```python
from build123d import *

# Parameters (mm, degrees)
F0_W     = 41
F0_H     = 106
F0_R     = 1.5
F0_R_2   = 5.05
F0_R_3   = 2
F0_R_4   = 3
F0_R_5   = 9.5
F1_DEPTH = 3
F2_R     = 3


# Not quite as in the source:
# - a feature names something its author has since deleted; it is built from what else it names


with BuildPart() as f1:
    # F0 (on Top) → F1 (new body)
    with BuildSketch(Plane.XY):
        with Locations((-1.1801278293, -1.1353523731)):
            Rectangle(F0_W, F0_H)
        with Locations((-18.2301278293, -51.4703523731)):
            Circle(F0_R, mode=Mode.SUBTRACT)
        with Locations((-6.776117335, -33.481924504)):
            Circle(F0_R_2, mode=Mode.SUBTRACT)
        with Locations((-18.2301278293, -21.2703523731)):
            Circle(F0_R, mode=Mode.SUBTRACT)
        with Locations((-11.8353097141, -18.4490393624)):
            Circle(F0_R_3, mode=Mode.SUBTRACT)
        with BuildLine():
            ThreePointArc((0.9913514778, -28.481924504), (-4.9415118708, -25.855220261), (-8.0481067447, -20.1589485871))
            Line((-8.0481067447, -20.1589485871), (9.9913514778, -20.516399593))
            Line((9.9913514778, -20.516399593), (9.9913514778, -46.516399593))
            Line((9.9913514778, -46.516399593), (-8.0481067447, -46.804900421))
            ThreePointArc((-8.0481067447, -46.804900421), (-4.9415118708, -41.1086287471), (0.9913514778, -38.481924504))
            Line((0.9913514778, -38.481924504), (0.9913514778, -28.481924504))
        make_face(mode=Mode.SUBTRACT)
        with Locations((15.0892422113, -51.4703523731)):
            Circle(F0_R, mode=Mode.SUBTRACT)
        with Locations((-1.1801278293, -10.9442314133)):
            Circle(F0_R_4, mode=Mode.SUBTRACT)
        with Locations((15.0892422113, -21.2703523731)):
            Circle(F0_R, mode=Mode.SUBTRACT)
        with Locations((-11.8353097141, -0.1353523731)):
            Circle(F0_R_3, mode=Mode.SUBTRACT)
        with Locations((-11.8353097141, 18.1783346161)):
            Circle(F0_R_3, mode=Mode.SUBTRACT)
        with Locations((-18.8301271707, 48.7366476269)):
            Circle(F0_R, mode=Mode.SUBTRACT)
        with Locations((-6.776117335, 33.2112197578)):
            Circle(F0_R_2, mode=Mode.SUBTRACT)
        with Locations((1.1698721707, 4.2646476269)):
            Circle(F0_R_5, mode=Mode.SUBTRACT)
        with BuildLine():
            ThreePointArc((0.9913514778, 38.2112197578), (-4.9415118708, 40.8379240009), (-8.0481067447, 46.5341956747))
            Line((-8.0481067447, 46.5341956747), (9.9913514778, 46.2456948468))
            Line((9.9913514778, 46.2456948468), (9.9913514778, 31.7237218389))
            ThreePointArc((9.9913514778, 31.7237218389), (10.4081379557, 31.2391097076), (10.6884153726, 30.6646495649))
            Line((10.6884153726, 30.6646495649), (12.8669505005, 24.7255908967))
            ThreePointArc((12.8669505005, 24.7255908967), (12.9813448828, 24.3018570593), (13.0198721707, 23.8646476269))
            ThreePointArc((13.0198721707, 23.8646476269), (12.0896967258, 21.9189727141), (9.9913514778, 21.4211530234))
            Line((9.9913514778, 21.4211530234), (9.9913514778, 20.2456948468))
            Line((9.9913514778, 20.2456948468), (-8.0481067447, 19.8882438409))
            ThreePointArc((-8.0481067447, 19.8882438409), (-4.9415118708, 25.5845155147), (0.9913514778, 28.2112197578))
            Line((0.9913514778, 28.2112197578), (0.9913514778, 38.2112197578))
        make_face(mode=Mode.SUBTRACT)
        with Locations((16.6392421771, 48.7366476269)):
            Circle(F0_R, mode=Mode.SUBTRACT)
        with BuildLine():
            Line((9.9913514778, -20.516399593), (-8.0481067447, -20.1589485871))
            ThreePointArc((-8.0481067447, -20.1589485871), (-4.9415118708, -25.855220261), (0.9913514778, -28.481924504))
            Line((0.9913514778, -28.481924504), (0.9913514778, -38.481924504))
            ThreePointArc((0.9913514778, -38.481924504), (-4.9415118708, -41.1086287471), (-8.0481067447, -46.804900421))
            Line((-8.0481067447, -46.804900421), (9.9913514778, -46.516399593))
            Line((9.9913514778, -46.516399593), (9.9913514778, -20.516399593))
        make_face()
        with Locations((-2.2937730764, -41.981924504)):
            Circle(F0_R, mode=Mode.SUBTRACT)
        with Locations((-2.2937730764, -24.981924504)):
            Circle(F0_R, mode=Mode.SUBTRACT)
        with BuildLine():
            Line((9.9913514778, 46.2456948468), (-8.0481067447, 46.5341956747))
            ThreePointArc((-8.0481067447, 46.5341956747), (-4.9415118708, 40.8379240009), (0.9913514778, 38.2112197578))
            Line((0.9913514778, 38.2112197578), (0.9913514778, 28.2112197578))
            ThreePointArc((0.9913514778, 28.2112197578), (-4.9415118708, 25.5845155147), (-8.0481067447, 19.8882438409))
            Line((-8.0481067447, 19.8882438409), (9.9913514778, 20.2456948468))
            Line((9.9913514778, 20.2456948468), (9.9913514778, 21.4211530234))
            ThreePointArc((9.9913514778, 21.4211530234), (8.9707387909, 21.9024586015), (8.2657292668, 22.7835186943))
            ThreePointArc((8.2657292668, 22.7835186943), (8.1741724057, 22.9999554201), (8.1033430916, 23.2240329142))
            Line((8.1033430916, 23.2240329142), (5.9741724057, 28.9999554201))
            ThreePointArc((5.9741724057, 28.9999554201), (6.9168863609, 31.9338578186), (9.9913514778, 31.7237218389))
            Line((9.9913514778, 31.7237218389), (9.9913514778, 46.2456948468))
        make_face()
        with Locations((-2.2937730764, 24.7112197578)):
            Circle(F0_R, mode=Mode.SUBTRACT)
        with Locations((-2.2937730764, 41.7112197578)):
            Circle(F0_R, mode=Mode.SUBTRACT)
        with Locations((-6.776117335, 33.2112197578)):
            Circle(F0_R_2)
        with Locations((-6.776117335, -33.481924504)):
            Circle(F0_R_2)
        with Locations((-11.8353097141, -18.4490393624)):
            Circle(F0_R_3)
        with Locations((-11.8353097141, -0.1353523731)):
            Circle(F0_R_3)
        with Locations((-11.8353097141, 18.1783346161)):
            Circle(F0_R_3)
        with Locations((-2.2937730764, -24.981924504)):
            Circle(F0_R)
        with Locations((-2.2937730764, -41.981924504)):
            Circle(F0_R)
        with Locations((-2.2937730764, 24.7112197578)):
            Circle(F0_R)
        with Locations((-2.2937730764, 41.7112197578)):
            Circle(F0_R)
    extrude(amount=F1_DEPTH)

    # F2
    f2_edges = [f1.edges().sort_by_distance(p)[0] for p in [
        (-21.680128, 51.864648, 1.5),
        (-21.680128, -54.135352, 1.5),
        (19.319872, -54.135352, 1.5),
        (19.319872, 51.864648, 1.5),
    ]]
    fillet(f2_edges, radius=F2_R)


solid = f1.part
```
Source: CAD feature listing. Evaluate the final solid. Frame: model axes, mm. A direction names the side the tool comes from. Round coordinates to 2 decimals unless told otherwise and drop trailing zeros. Loops run counter-clockwise (first coordinate to the right, second up) from the corner with the lowest first, then second, coordinate; pieces in that order, holes last. Notation, with made-up numbers: M 10,12.5 L 34,12.5 A21 ccw 34,26.5 Z; hole C -21.5,44 d10. An arc over 180 degrees is marked long. Use a Markdown table: item, result. Add a question column.
1. Cut plane B-B, the plane y = -13. Output: boundary loops of the cut face in (x, z), and give its area (3 significant figures).
2. Contact query for a flat-ended pin moving along its axis: pin 1 (5 mm diameter, centred on x = -18.23, y = -51.47, fed in from -Z). Output: stop coordinate, or through.
3. Ray query, line 1 along Y through (x, z) = (-1, 0.6); line 2 along Y through (x, z) = (-19.5, 1.35); line 3 along Y through (x, z) = (-1.5, 0.65). Return the intervals inside material, ascending. Write a range as [from, to].
4. Set-up query: faces 1 (the flat face through (7.054, 26.072, 1.479)), 2 (the cylindrical face through (18.42, -53.28, 1.52)). Return all of +Z, -Z, +X, -X, +Y, -Y with unobstructed straight access to the full face (end or side cutting, diameter ignored); none if empty.
5. Cut plane A-A, the plane z = 2.2. State how many separate pieces and enclosed holes the cut face has, and give its area (3 significant figures).
6. Pull-direction query (X, two-part tool) for faces 3 (the flat face through (19.32, -2, 1)), 4 (the flat face through (-1, 51.865, 1)), 5 (the cylindrical face through (15.9, -50.21, 1.48)); classes: +X half, -X half, draft (parallel to the pull), parting line (faces both ways), or undercut.
7. Cut plane C-C, the plane x = 3. Output: boundary loops of the cut face in (y, z), and give its area (3 significant figures).
Solution:
| question | item | result |
|---|---|---|
| 1 | outline | M -21.68,0 L -3.37,0 L -3.37,3 L -21.68,3 Z; M 1,0 L 19.32,0 L 19.32,3 L 1,3 Z |
| 1 | area | 110 mm2 |
| 2 | pin 1 | stops at z = 0 |
| 3 | line 1 | y = [-54.14, -13.94], [-7.95, -4.98], [13.51, 51.86] |
| 3 | line 2 | y = [-54.02, -52.27], [-50.67, -22.07], [-20.47, 47.39], [50.08, 51.75] |
| 3 | line 3 | y = [-54.14, -13.93], [-7.96, -4.85], [13.38, 51.86] |
| 4 | face 1 | +Z, -Z |
| 4 | face 2 | +Z, -Z, +X, -Y |
| 5 | separate pieces | 1 |
| 5 | enclosed holes | 9 |
| 5 | area | 3,930 mm2 |
| 6 | face 3 | +X half |
| 6 | face 4 | draft |
| 6 | face 5 | undercut |
| 7 | outline | M -54.14,0 L -5.06,0 L -5.06,3 L -54.14,3 Z; M 13.59,0 L 51.86,0 L 51.86,3 L 13.59,3 Z |
| 7 | area | 262 mm2 |
